Design review of the part shown in the three views and the two pictorial views. Dimensions are in mm from the part's minimum x, y and z. A direction names the side the tool comes from. Coordinates: 2 decimals unless noted, no trailing zeros. Loops run counter-clockwise (first coordinate to the right, second up) from the corner with the lowest first, then second, coordinate; pieces in that order, holes last.
Q1. Add section B-B on z = 162. Give the boundary of the cut face in (x, y), and give its area (3 significant figures).
Q2. For P1, Ø16.5, axis at y = 114.5, z = 177.5, coming from the -X side, flat-tipped, find the tip position at first contact; note if it passes through.
Q3. Machinability: for the marked faces 1, 2 and 3, which of the approach directions +Z, -Z, +X, -X, +Y, -Y give a long, thin tool a straight path to every point of the face, cutting with its end or side? Answer none if there is none.
Q4. Add section A-A on x = 107. Give the boundary of the cut face in (y, z).
Q5. Add section C-C on y = 77.5. Give the boundary of the cut face in (x, z), and give its area (4 significant figures).
Q6. Add section D-D on x = 56. Give the boundary of the cut face in (y, z).
Q7. Wall thickness on probe 1 along Y at (x, z) = (51, 190.5); probe 2 along X at (y, z) = (178, 101); probe 3 along X at (y, z) = (113, 174.5): over which ranges is each line inside the solid? List them lowest first.
Q8. Draft analysis for pull direction Y (two halves, no side actions). For the marked faces 4, 5 and 6, state which applies: released by +Y, released by -Y, zero draft, split by the parting line, or undercut.
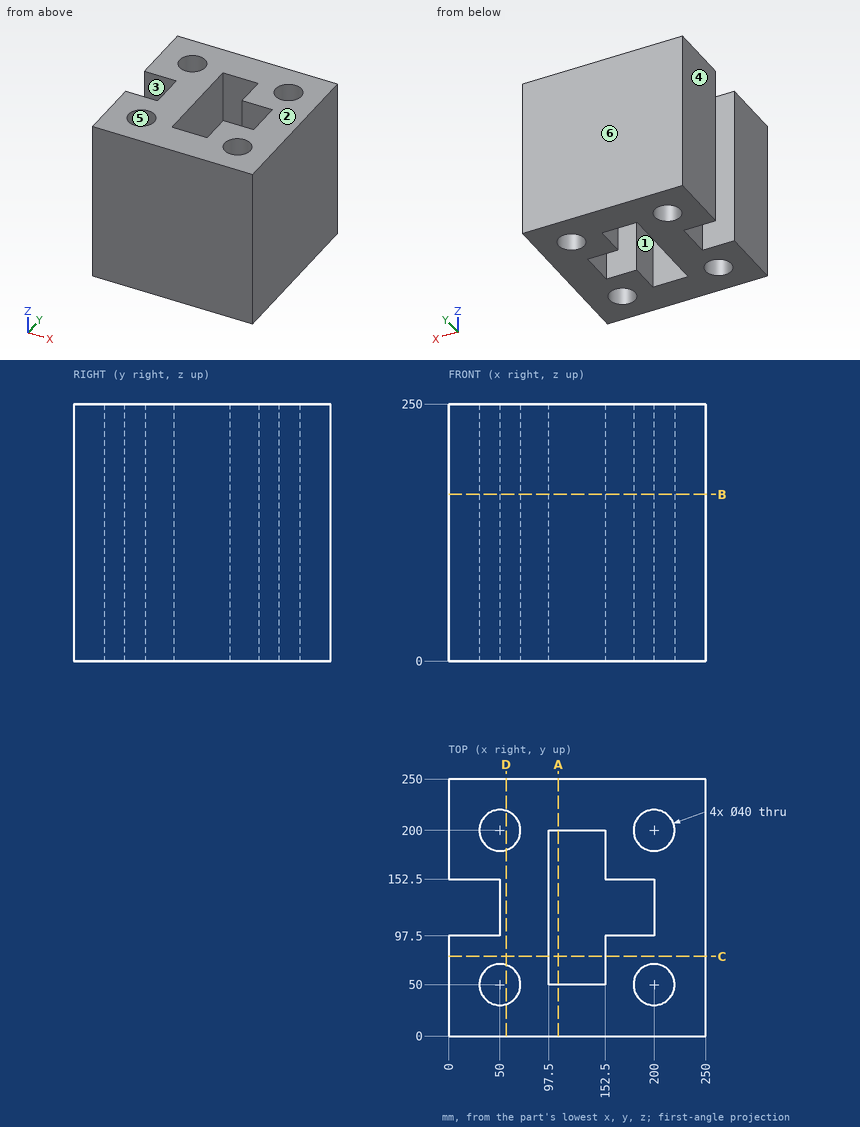
Entries:
1. outline: (0, 0) - (250, 0) - (250, 250) - (0, 250) - (0, 152.5) - (50, 152.5) - (50, 97.5) - (0, 97.5) - close; hole circle Ø40 at (50, 50); hole circle Ø40 at (50, 200); hole (97.5, 50) - (152.5, 50) - (152.5, 97.5) - (200, 97.5) - (200, 152.5) - (152.5, 152.5) - (152.5, 200) - (97.5, 200) - close; hole circle Ø40 at (200, 50); hole circle Ø40 at (200, 200)
1. area: 43,900 mm2
2. P1: stops at x = 50
3. face 1: +Z, -Z
3. face 2: +Z, +X, -X, +Y, -Y
3. face 3: +Z, -Z, -X
4. outline: (0, 0) - (50, 0) - (50, 250) - (0, 250) - close; (200, 0) - (250, 0) - (250, 250) - (200, 250) - close
5. outline: (0, 0) - (97.5, 0) - (97.5, 250) - (0, 250) - close; (152.5, 0) - (250, 0) - (250, 250) - (152.5, 250) - close
5. area: 48,750 mm2
6. outline: (0, 0) - (30.92, 0) - (30.92, 250) - (0, 250) - close; (69.08, 0) - (180.92, 0) - (180.92, 250) - (69.08, 250) - close; (219.08, 0) - (250, 0) - (250, 250) - (219.08, 250) - close
7. probe 1: y = 0 to 30.03, 69.97 to 180.03, 219.97 to 250
7. probe 2: x = 0 to 97.5, 152.5 to 250
7. probe 3: x = 50 to 97.5, 200 to 250
8. face 4: zero draft
8. face 5: undercut
8. face 6: released by +Y
